Solid Edge part; units mm, degrees
sketch "Sketch1" plane through (0, 0, 0) normal (0, -1, 0) x (1, 0, 0)
  arc A0 (0, 0) -> (8, 8) centre (0, 8) cw
  line L0 (8, 8) -> (8, 6)
  line L1 (8, 6) -> (48, 6)
  arc A1 (48, 6) -> (50, 4) centre (48, 4) cw
  line L2 (50, 4) -> (50, 0)
  line L3 (50, 0) -> (0, 0)
extrude "ExtrudedProtrusion_1" add sketch "Sketch1" against normal blind 62.5 and the other way blind 62.5
sketch "Sketch2" plane through (0, 0, 0) normal (0, 0, 1) x (1, 0, 0)
  line L0 (-21, 62.5) -> (-21, -62.5)
  line L1 (-21, -62.5) -> (8.3, -62.5)
  line L2 (8.3, -62.5) -> (8.3, -36.8)
  line L3 (8.3, -36.8) -> (-16, -36.8)
  line L4 (-16, -36.8) -> (-16, -13.2)
  line L5 (-16, -13.2) -> (8.3, -13.2)
  line L6 (8.3, -13.2) -> (8.3, 13.2)
  line L7 (8.3, 13.2) -> (-16, 13.2)
  line L8 (-16, 13.2) -> (-16, 36.8)
  line L9 (-16, 36.8) -> (8.3, 36.8)
  line L10 (8.3, 36.8) -> (8.3, 62.5)
  line L11 (8.3, 62.5) -> (-21, 62.5)
extrude "ExtrudedCutout_1" cut sketch "Sketch2" along normal blind 16
sketch "Sketch3" plane through (30, 0, 0) normal (1, 0, 0) x (0, 1, 0)
  line L0 (37.5, 6) -> (43.8, 6)
  line L1 (43.8, 6) -> (40.8, 3)
  line L2 (40.8, 3) -> (40.8, 0)
  line L3 (40.8, 0) -> (37.5, 0)
  line L4 (37.5, 0) -> (37.5, 6)
revolve "RevolvedCutout1" cut sketch "Sketch3" angle 360 about axis through (30, 37.5, 0) along (0, 0, 1)
sketch "Sketch4" plane through (30, 0, 0) normal (1, 0, 0) x (0, 1, 0)
  line L0 (-37.5, 6) -> (-31.2, 6)
  line L1 (-31.2, 6) -> (-34.2, 3)
  line L2 (-34.2, 3) -> (-34.2, 0)
  line L3 (-34.2, 0) -> (-37.5, 0)
  line L4 (-37.5, 0) -> (-37.5, 6)
revolve "RevolvedCutout2" cut sketch "Sketch4" angle 360 about axis through (30, -37.5, 0) along (0, 0, 1)
sketch "Sketch5" plane through (30, 0, 0) normal (1, 0, 0) x (0, 1, 0)
  line L0 (0, 6) -> (6.3, 6)
  line L1 (6.3, 6) -> (3.3, 3)
  line L2 (3.3, 3) -> (3.3, 0)
  line L3 (3.3, 0) -> (0, 0)
  line L4 (0, 0) -> (0, 6)
revolve "RevolvedCutout3" cut sketch "Sketch5" angle 360 about axis through (30, 0, 0) along (0, 0, 1)
sketch "Sketch6" plane through (0, 0, 0) normal (1, 0, 0) x (0, 1, 0)
  arc A0 (-60.5, 8) -> (-56.5, 12) centre (-56.5, 8) cw
  line L0 (-56.5, 12) -> (56.5, 12)
  arc A1 (56.5, 12) -> (60.5, 8) centre (56.5, 8) cw
  line L1 (60.5, 8) -> (-60.5, 8)
revolve "RevolvedCutout4" cut sketch "Sketch6" angle 360 about axis through (0, 60.5, 8) along (0, -1, 0)
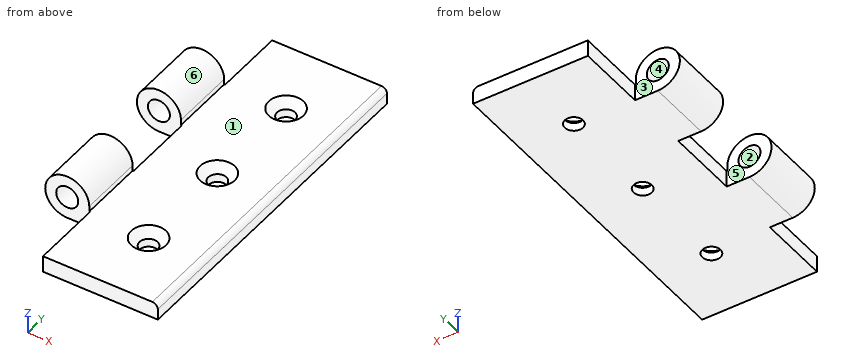
Part model, mm, in its own coordinate system. Face numbers are marked on the shaded views. A direction names the side the tool comes from. Coordinates: 2 decimals unless noted, no trailing zeros. Order: outer loops, then holes, each group sorted by start corner. A loop starts at its lowest first (then second) coordinate and runs counter-clockwise, first axis right, second up.
(1) Probe L1, parallel to Y at x = 30, z = 1; L2, parallel to X at y = 0, z = 2.05; L3, parallel to Y at x = 4.5, z = 12.75. List the from-to ranges inside material, lowest first.
Check sheet entries:
L1: y = -62.5 to -40.8, -34.2 to -3.3, 3.3 to 34.2, 40.8 to 62.5
L2: x = 8.3 to 26.7, 33.3 to 50
L3: y = -36.8 to -13.2, 13.2 to 36.8
(2) Slice it at A-A, the plane x = 30. Write the cut outline in (y, z), and give its area (3 significant figures).
Check sheet entries:
outline: (-62.5, 0) - (-40.8, 0) - (-40.8, 3) - (-43.8, 6) - (-62.5, 6) - close; (-34.2, 0) - (-3.3, 0) - (-3.3, 3) - (-6.3, 6) - (-31.2, 6) - (-34.2, 3) - close; (3.3, 0) - (34.2, 0) - (34.2, 3) - (31.2, 6) - (6.3, 6) - (3.3, 3) - close; (40.8, 0) - (62.5, 0) - (62.5, 6) - (43.8, 6) - (40.8, 3) - close
area: 604 mm2
(3) Pin check, flat tips, straight feed: pin 1 Ø5 at (x, z) = (-2.5, 8.5) entering from +Y; pin 2 Ø2 at (y, z) = (-25.5, 7.5) entering from +X; pin 3 Ø6 at (x, y) = (29, -2) entering from -Z; pin 4 Ø5 at (x, y) = (43.5, 12) entering from +Z. Stop position of each tip, or through.
Check sheet entries:
pin 1: stops at y = 36.8
pin 2: stops at x = 8
pin 3: stops at z = 0
pin 4: stops at z = 6
(4) Slice it at D-D, the plane y = 0. Write the cut outline in (x, z).
Check sheet entries:
outline: (8.3, 0) - (26.7, 0) - (26.7, 3) - (23.7, 6) - (8.3, 6) - close; (33.3, 0) - (50, 0) - (50, 4) arc R2 ccw to (48, 6) - (36.3, 6) - (33.3, 3) - close
(5) Slice it at B-B, the plane y = -17.5. Write the cut outline in (x, z), and give its area (3 significant figures).
Check sheet entries:
outline: (0, 0) - (50, 0) - (50, 4) arc R2 ccw to (48, 6) - (8, 6) - (8, 8) arc R8 ccw (long way) to start; hole circle Ø8 at (0, 8)
area: 416 mm2
(6) Tool access for the marked faces 1, 2 and 3: list every direction of +Z, -Z, +X, -X, +Y, -Y with a clear straight run to the whole face (end or side of a thin tool).
Check sheet entries:
face 1: +Z, +X, +Y, -Y
face 2: +Y, -Y
face 3: +Z, -Z, -X, +Y
(7) Slice it at C-C, the plane z = 9.25. Write the cut outline in (x, y), and give its area (3 significant figures).
Check sheet entries:
outline: (-7.9, -36.8) - (-3.8, -36.8) - (-3.8, -13.2) - (-7.9, -13.2) - close; (-7.9, 13.2) - (-3.8, 13.2) - (-3.8, 36.8) - (-7.9, 36.8) - close; (3.8, -36.8) - (7.9, -36.8) - (7.9, -13.2) - (3.8, -13.2) - close; (3.8, 13.2) - (7.9, 13.2) - (7.9, 36.8) - (3.8, 36.8) - close
area: 387 mm2
(8) Pull direction Z, two halves, no side cores. Call the marked faces 4, 5 and 6: pulls with the +Z half, pulls with the -Z half, needs draft (parallel to the pull), parting line crosses it, or undercut.
Check sheet entries:
face 4: undercut
face 5: needs draft
face 6: parting line crosses it
